Geometry check sheet. Reference: the model listing, model coordinates, mm. Face numbers are marked on the shaded views. Round coordinates to 2 decimals unless told otherwise and drop trailing zeros. Write each loop counter-clockwise with the first axis right and the second up, starting at its lowest first coordinate (ties: lowest second). Pieces come first, ordered by that corner, then holes. Notation, with made-up numbers: (-17.75, 54.25) -> (29.25, 54.25) arc R28 cw to (29.25, 78.25) -> close; hole circle Ø9 at (86.5, 5). An arc over 180 degrees is marked (long way). One line per question, with ' | ' between items.
```python
from build123d import *

# Parameters (mm, degrees)
F1_DEPTH = 9.525


# Not quite as in the source:
# - a length typed as a fraction of an inch, garbled in the dataset ("3 / 203.2 mm" for 3/8 in), is restored


with BuildPart() as f1:
    # F0 (on Top) → F1 (new body)
    with BuildSketch(Plane.XY):
        with BuildLine():
            ThreePointArc((0, 27.0671695471), (-4.5048536548, 25.1556778504), (-8.2258973271, 21.977417171))
            ThreePointArc((-8.2258973271, 21.977417171), (-9.7181261566, 18.698842434), (-9.2097157612, 15.1327075437))
            ThreePointArc((-9.2097157612, 15.1327075437), (-10.6205392688, 11.8246856933), (-10.2093555033, 8.2519613206))
            Line((-10.2093555033, 8.2519613206), (-12.369341217, 7.1464567445))
            Line((-12.369341217, 7.1464567445), (-12.369341217, 4.6386048198))
            Line((-12.369341217, 4.6386048198), (-12.369341217, 4.5682978211))
            ThreePointArc((-12.369341217, 4.5682978211), (-15.5930977879, 3.1185654947), (-17.7027139134, 0.2823972963))
            ThreePointArc((-17.7027139134, 0.2823972963), (-21.0452825194, -1.0603738309), (-23.1384971151, -3.9919692741))
            ThreePointArc((-23.1384971151, -3.9919692741), (-26.5647165348, -5.2934051439), (-28.80180468, -8.19653302))
            ThreePointArc((-28.80180468, -8.19653302), (-29.7673344436, -12.5572908836), (-29.5614041388, -17.0189104974))
            ThreePointArc((-29.5614041388, -17.0189104974), (-25.7783661022, -19.4669407743), (-21.4921734029, -20.8571857766))
            ThreePointArc((-21.4921734029, -20.8571857766), (-17.8594468391, -20.3713745504), (-15.0192606046, -18.054899429))
            ThreePointArc((-15.0192606046, -18.054899429), (-11.4338171794, -17.7079201351), (-8.5996589687, -15.484556372))
            ThreePointArc((-8.5996589687, -15.484556372), (-5.0294162563, -15.0523544446), (-2.1409380715, -12.9098966718))
            Line((-2.1409380715, -12.9098966718), (0, -14.2561570176))
            Line((0, -14.2561570176), (1.9696742658, -12.9098966718))
            ThreePointArc((1.9696742658, -12.9098966718), (4.9392756736, -15.0084468105), (8.560301624, -15.3410370587))
            ThreePointArc((8.560301624, -15.3410370587), (11.3944598347, -17.5644008218), (14.9799032599, -17.9113801157))
            ThreePointArc((14.9799032599, -17.9113801157), (17.8200894944, -20.2278552371), (21.4528160582, -20.7136664634))
            ThreePointArc((21.4528160582, -20.7136664634), (25.6558468929, -19.2922500665), (29.4813849032, -17.0447733253))
            ThreePointArc((29.4813849032, -17.0447733253), (29.5836204245, -12.511977875), (28.7624473353, -8.0530137067))
            ThreePointArc((28.7624473353, -8.0530137067), (26.5253591901, -5.1498858306), (23.0991397704, -3.8484499608))
            ThreePointArc((23.0991397704, -3.8484499608), (21.0059251747, -0.9168545176), (17.6633565687, 0.4259166096))
            ThreePointArc((17.6633565687, 0.4259166096), (15.4847616458, 3.3168082822), (12.1560195839, 4.739132713))
            Line((12.1560195839, 4.739132713), (12.1560195839, 7.1464567445))
            Line((12.1560195839, 7.1464567445), (9.9960338703, 8.2519613206))
            ThreePointArc((9.9960338703, 8.2519613206), (10.4072176357, 11.8246856933), (8.9963941282, 15.1327075437))
            ThreePointArc((8.9963941282, 15.1327075437), (9.5048045235, 18.698842434), (8.012575694, 21.977417171))
            ThreePointArc((8.012575694, 21.977417171), (4.4155385291, 25.1665589), (0, 27.0671695471))
        make_face()
    extrude(amount=F1_DEPTH)


solid = f1.part
```
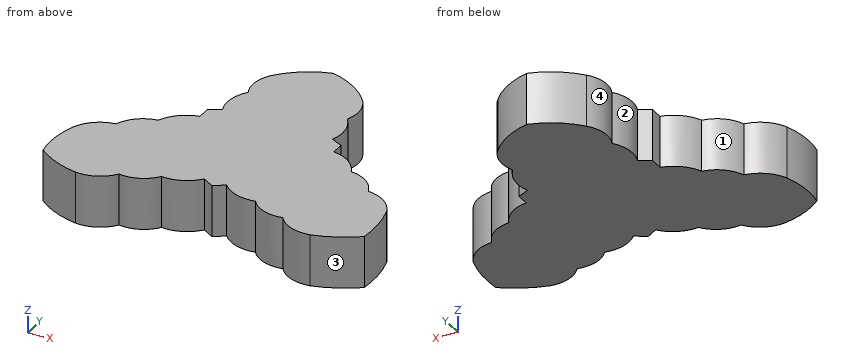
(1) Go/stop test with flat-tipped pins: pin 1 (2 mm diameter, centred on y = -8, z = 2.5, fed in from -X); pin 2 (2 mm diameter, centred on y = 6.5, z = 5, fed in from +X); pin 3 (2 mm diameter, centred on y = 6, z = 7, fed in from -X). Record where each tip stops, or that it passes through.
Resolved:
pin 1: stops at x = -29.07 | pin 2: stops at x = 12.16 | pin 3: stops at x = -12.37
(2) Sectioned sample at C-C on x = -3.5. Record the cut outline in (y, z) (1 decimal), then the cut area to 3 significant figures.
Resolved:
outline: (-14.2, 0) -> (25.7, 0) -> (25.7, 9.5) -> (-14.2, 9.5) -> close | area: 380 mm2
(3) Sectioned sample at B-B on y = -5.5. Record the cut outline in (x, z) (3 decimals).
Resolved:
outline: (-26.829, 0) -> (26.958, 0) -> (26.958, 9.525) -> (-26.829, 9.525) -> close
(4) Draft check along Y on the marked faces 1, 2, 3 and 4. Enter one of: +Y half, -Y half, draft (parallel to the pull), parting line (faces both ways), or undercut.
Resolved:
face 1: +Y half | face 2: undercut | face 3: -Y half | face 4: undercut
(5) Sectioned sample at A-A on z = 8.75. Record the cut outline in (x, y).
Resolved:
outline: (-29.56, -17.02) arc R17.33 ccw to (-21.49, -20.86) arc R6.73 ccw to (-15.02, -18.05) arc R6.42 ccw to (-8.6, -15.48) arc R7.02 ccw to (-2.14, -12.91) -> (0, -14.26) -> (1.97, -12.91) arc R7.02 ccw to (8.56, -15.34) arc R6.42 ccw to (14.98, -17.91) arc R6.73 ccw to (21.45, -20.71) arc R21.68 ccw to (29.48, -17.04) arc R22.19 ccw to (28.76, -8.05) arc R6.73 ccw to (23.1, -3.85) arc R6.42 ccw to (17.66, 0.43) arc R7.02 ccw to (12.16, 4.74) -> (12.16, 7.15) -> (10, 8.25) arc R7.02 ccw to (9, 15.13) arc R6.42 ccw to (8.01, 21.98) arc R15.14 ccw to (0, 27.07) arc R16.08 ccw to (-8.23, 21.98) arc R6.42 ccw to (-9.21, 15.13) arc R7.02 ccw to (-10.21, 8.25) -> (-12.37, 7.15) -> (-12.37, 4.57) arc R7.02 ccw to (-17.7, 0.28) arc R6.42 ccw to (-23.14, -3.99) arc R6.73 ccw to (-28.8, -8.2) arc R16.97 ccw to start
(6) Material ranges on line 1 (X direction, y = -14, z = 8.25); line 2 (X direction, y = 7, z = 3.25); line 3 (Y direction, x = -26, z = 3.75), recorded low to high.
Resolved:
line 1: x = -29.83 to -3.23, -0.41 to 0.37, 3.11 to 29.65 | line 2: x = -12.37 to 12.16 | line 3: y = -19.36 to -4.92
